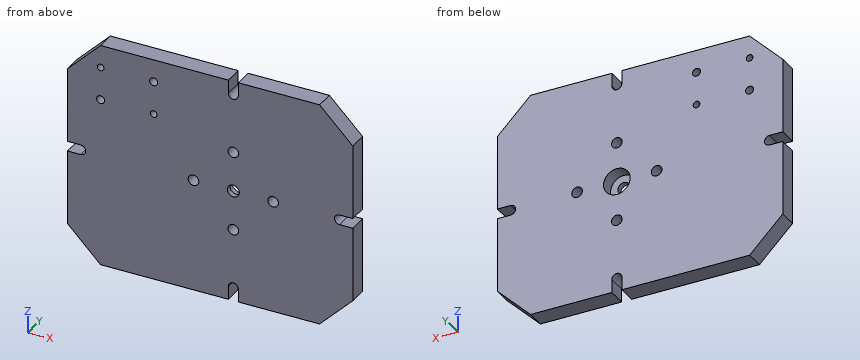
from build123d import *

# Parameters (mm, degrees)
EXTRUDE_1_DEPTH     = 28
SKETCH_2_R          = 8
CUT_EXTRUDE_1_DEPTH = 28
SKETCH_3_R          = 6
SKETCH_3_R_2        = 5
CUT_EXTRUDE_2_DEPTH = 28
SKETCH_4_R          = 20
CUT_EXTRUDE_3_DEPTH = 20
SKETCH_5_R          = 9
CUT_EXTRUDE_4_DEPTH = 20


with BuildPart() as part:
    # Эскиз1 → Бобышка-Вытянуть1 (new body)
    with BuildSketch(Plane(origin=(0, 0, 0), x_dir=(1, 0, 0), z_dir=(0, 1, 0))):
        with BuildLine():
            Line((0, 50), (50, 0))
            Line((50, 0), (242.5, 0))
            Line((242.5, 0), (242.5, 20))
            ThreePointArc((242.5, 20), (250, 27.5), (257.5, 20))
            Line((257.5, 20), (257.5, 0))
            Line((257.5, 0), (380, 0))
            Line((380, 0), (430, 50))
            Line((430, 50), (430, 162.5))
            Line((430, 162.5), (410, 162.5))
            ThreePointArc((410, 162.5), (402.5, 170), (410, 177.5))
            Line((410, 177.5), (430, 177.5))
            Line((430, 177.5), (430, 290))
            Line((430, 290), (380, 340))
            Line((380, 340), (257.5, 340))
            Line((257.5, 340), (257.5, 320))
            ThreePointArc((257.5, 320), (250, 312.5), (242.5, 320))
            Line((242.5, 320), (242.5, 340))
            Line((242.5, 340), (50, 340))
            Line((50, 340), (0, 290))
            Line((0, 290), (0, 177.5))
            Line((0, 177.5), (20, 177.5))
            ThreePointArc((20, 177.5), (27.5, 170), (20, 162.5))
            Line((20, 162.5), (0, 162.5))
            Line((0, 162.5), (0, 50))
        make_face()
    extrude(amount=EXTRUDE_1_DEPTH)

    # Эскиз2 → Вырез-Вытянуть1 (cut)
    with BuildSketch(Plane(origin=(0, 28, 0), x_dir=(1, 0, 0), z_dir=(0, 1, 0))):
        with Locations((250, 230)):
            Circle(SKETCH_2_R)
        with Locations((190, 170)):
            Circle(SKETCH_2_R)
        with Locations((250, 110)):
            Circle(SKETCH_2_R)
        with Locations((310, 170)):
            Circle(SKETCH_2_R)
    extrude(amount=-CUT_EXTRUDE_1_DEPTH, mode=Mode.SUBTRACT)

    # Эскиз3 → Вырез-Вытянуть2 (cut)
    with BuildSketch(Plane(origin=(0, 28, 0), x_dir=(1, 0, 0), z_dir=(0, 1, 0))):
        with Locations((50, 84)):
            Circle(SKETCH_3_R)
        with Locations((130, 84)):
            Circle(SKETCH_3_R_2)
        with Locations((50, 34)):
            Circle(SKETCH_3_R_2)
        with Locations((130, 34)):
            Circle(SKETCH_3_R)
    extrude(amount=-CUT_EXTRUDE_2_DEPTH, mode=Mode.SUBTRACT)

    # Эскиз4 → Вырез-Вытянуть3 (cut)
    with BuildSketch(Plane(origin=(0, 28, 0), x_dir=(1, 0, 0), z_dir=(0, 1, 0))):
        with Locations((250, 170)):
            Circle(SKETCH_4_R)
    extrude(amount=-CUT_EXTRUDE_3_DEPTH, mode=Mode.SUBTRACT)

    # Эскиз5 → Вырез-Вытянуть4 (cut)
    with BuildSketch(Plane(origin=(0, 8, 0), x_dir=(1, 0, 0), z_dir=(0, 1, 0))):
        with Locations((250, 170)):
            Circle(SKETCH_5_R)
    extrude(amount=-CUT_EXTRUDE_4_DEPTH, mode=Mode.SUBTRACT)


solid = part.part
Geometry: final body of the model. Coordinates: model frame, mm. Coordinates: 2 decimals unless noted, no trailing zeros. Order: outer loops, then holes, each group sorted by start corner. A loop starts at its lowest first (then second) coordinate and runs counter-clockwise, first axis right, second up.
(1) Section query B-B (y = 18). State how many separate pieces and enclosed holes the cut face has, plus the area to 3 significant figures.
(2) Section query C-C (x = 310). Return the cut outline in (y, z), plus the area to 3 significant figures.
(3) First-contact query: pin 1 (6 mm diameter, centred on y = 15, z = -331.5, fed in from -X); pin 2 (16 mm diameter, centred on x = 421, y = 19, fed in from +Z); pin 3 (16 mm diameter, centred on y = 7.5, z = -8, fed in from +X). Flat tips, straight axial feed; report the tip coordinate or a pass-through.
(4) Section query D-D (z = -230). Return the cut outline in (x, y), plus the area to 3 significant figures.
(5) Section query A-A (x = 130). Return the cut outline in (y, z), plus the area to 3 significant figures.
(6) Material intervals for probe 1 along Z at (x, y) = (250, 9.75); probe 2 along Z at (x, y) = (130, 10); probe 3 along X at (y, z) = (15, -110), sorted ascending.
Solution:
1. separate pieces: 1
1. enclosed holes: 9
1. area: 137,000 mm2
2. outline: (0, -340) - (28, -340) - (28, -178) - (0, -178) - close; (0, -162) - (28, -162) - (28, 0) - (0, 0) - close
2. area: 9,070 mm2
3. pin 1: stops at x = 38.5
3. pin 2: stops at z = -33
3. pin 3: stops at x = 396
4. outline: (0, 0) - (242, 0) - (242, 28) - (0, 28) - close; (258, 0) - (430, 0) - (430, 28) - (258, 28) - close
4. area: 11,600 mm2
5. outline: (0, -340) - (28, -340) - (28, -89) - (0, -89) - close; (0, -79) - (28, -79) - (28, -40) - (0, -40) - close; (0, -28) - (28, -28) - (28, 0) - (0, 0) - close
5. area: 8,900 mm2
6. probe 1: z = -312.5 to -238, -222 to -190, -150 to -118, -102 to -27.5
6. probe 2: z = -340 to -89, -79 to -40, -28 to 0
6. probe 3: x = 0 to 242, 258 to 430
